from build123d import *

# Parameters (mm, degrees)
HEXAGONSOCKET_DEPTH = 1.1
CHAMFER_2_SIZE      = 0.2705
SKETCH_1_R          = 3.36
EXTRUDE_4_DEPTH     = 0.5
EXTRUDE_START       = 0.15
SKETCH_8_R          = 3.36
EXTRUDE_6_DEPTH     = 0.15
FILLET_5_R          = 0.2
CUT_EXTRUDE_START   = 3.14
SKETCH_6_R          = 1.5
CUT_EXTRUDE_1_DEPTH = 5.628101593
FILLET_6_R          = 0.15
CHAMFER_1_SIZE      = 0.15


with BuildPart() as part:
    # Sketch1 → Base (revolve)
    with BuildSketch(Plane.XY, mode=Mode.PRIVATE) as base_sk:
        Polygon((0, 0), (0, 3.36), (1.86, 1.5), (8, 1.5), (8, 0), align=None)
    revolve(base_sk.sketch.rotate(Axis((-0.587069181, 0, 0), (1, 0, 0)), 90), axis=Axis((-0.587069181, 0, 0), (1, 0, 0)))

    # Sketch2 → HexagonSocket (cut)
    with BuildSketch(Plane(origin=(0, 0, 0), x_dir=(0, 0, -1), z_dir=(1, 0, 0))):
        Polygon((1.154700538, 0), (0.577350269, 1), (-0.577350269, 1), (-1.154700538, 0), (-0.577350269, -1), (0.577350269, -1), align=None)
    extrude(amount=HEXAGONSOCKET_DEPTH, mode=Mode.SUBTRACT)

    # Sketch3 → Cut-Revolve1 (revolve, cut)
    with BuildSketch(Plane.XY, mode=Mode.PRIVATE) as cut_revolve1_sk:
        Polygon((1.1, 1), (1.677350269, 0), (1.1, 0), align=None)
    revolve(cut_revolve1_sk.sketch.rotate(Axis((-0.439109555, 0, 0), (1, 0, 0)), 90), axis=Axis((-0.439109555, 0, 0), (1, 0, 0)), mode=Mode.SUBTRACT)

    # Chamfer 2
    chamfer_2_edges = [part.edges().sort_by_distance(p)[0] for p in [
        (8, 0, -1.5),
    ]]
    chamfer(chamfer_2_edges, length=CHAMFER_2_SIZE)

    # 草图1 → 凸台-拉伸4 (add)
    with BuildSketch(Plane.ZY):
        Circle(SKETCH_1_R)
        Polygon((0.577350269, -1), (-0.577350269, -1), (-1.154700538, 0), (-0.577350269, 1), (0.577350269, 1), (1.154700538, 0), align=None, mode=Mode.SUBTRACT)
    extrude(amount=-EXTRUDE_4_DEPTH)

    # 草图5 → 旋转7 (revolve)
    with BuildSketch(Plane(origin=(0, 0, 0), x_dir=(1, 0, 0), z_dir=(0, 0.5000000000000003, 0.8660254037844386)), mode=Mode.PRIVATE) as revolve_7_sk:
        Polygon((2.632985321, -0.645763152), (0.5, -2.778748473), (0.5, -3.36), (2.632985321, -1.227014679), align=None)
    revolve(revolve_7_sk.sketch.rotate(Axis((1.86, 0, 0), (-1, 0, 0)), 60), axis=Axis((1.86, 0, 0), (-1, 0, 0)))

    # 草图8 → 凸台-拉伸6 (add)
    with BuildSketch(Plane.ZY.offset(EXTRUDE_START)):
        Circle(SKETCH_8_R)
        Polygon((0.577350269, -1), (-0.577350269, -1), (-1.154700538, 0), (-0.577350269, 1), (0.577350269, 1), (1.154700538, 0), align=None, mode=Mode.SUBTRACT)
    extrude(amount=-EXTRUDE_6_DEPTH)

    # 草图11 → 旋转8 (revolve)
    with BuildSketch(Plane(origin=(0, 0, 0), x_dir=(1, 0, 0), z_dir=(0, 0.5000000000000003, 0.8660254037844386)), mode=Mode.PRIVATE) as revolve_8_sk:
        Polygon((0.5, -3.36), (0.217401845, -3.642598155), (0, -3.86), (-0.15, -3.71), (-0.15, -3.36), align=None)
    revolve(revolve_8_sk.sketch.rotate(Axis((-0.15, 0, 0), (1, 0, 0)), 300), axis=Axis((-0.15, 0, 0), (1, 0, 0)))

    # 圆角5
    fillet_5_edges = [part.edges().sort_by_distance(p)[0] for p in [
        (0, 0, -3.86),
    ]]
    fillet(fillet_5_edges, radius=FILLET_5_R)

    # 草图6 → 切除-拉伸1 (cut, through all)
    with BuildSketch(Plane(origin=(2.36, 0, 0), x_dir=(0, 0, -1), z_dir=(1, 0, 0)).offset(CUT_EXTRUDE_START)):
        with Locations(Location((0, 0, 0), (0, 0, 180))):
            Circle(SKETCH_6_R)
    extrude(amount=CUT_EXTRUDE_1_DEPTH, mode=Mode.SUBTRACT)

    # 圆角6
    fillet_6_edges = [part.edges().sort_by_distance(p)[0] for p in [
        (2.36, 0, -1.5),
    ]]
    fillet(fillet_6_edges, radius=FILLET_6_R)

    # 倒角1
    chamfer_1_edges = [part.edges().sort_by_distance(p)[0] for p in [
        (5.5, 0, -1.5),
    ]]
    chamfer(chamfer_1_edges, length=CHAMFER_1_SIZE)


solid = part.part
Input: part model. Units: mm. Frame: model coordinates. Give positions to 0.01 mm unless a question says otherwise; leave off trailing zeros. Write each loop counter-clockwise with the first axis right and the second up, starting at its lowest first coordinate (ties: lowest second). Pieces come first, ordered by that corner, then holes. Notation, with made-up numbers: (-33.75, 78) -> (-27.75, 78) arc R8 cw to (-27.75, 84) -> close; hole circle Ø11 at (42.5, -9). An arc over 180 degrees is marked (long way). Use one line per item in the form item = value. Start each with the question number.
1) Draft query along Z for faces 1 (the flat face through (0.5, -1, 0)), 2 (the cylindrical face through (3.91, -0.45, 1.43)), 3 (the flat face through (5.5, 0, 0)). Return one class per face: pulls with the +Z half, pulls with the -Z half, needs draft (parallel to the pull), parting line crosses it, or undercut.
2) Pin query (flat end, axial travel): pin 1 (3 mm diameter, centred on x = 2.5, z = 1.5, fed in from -Y); pin 2 (2 mm diameter, centred on x = 4.5, y = -1.5, fed in from -Z); pin 3 (0.9 mm diameter, centred on x = 0.5, z = 0, fed in from -Y). Return the tip coordinate at first contact, or that it passes through.
3) Section query C-C on x = 4.8. Return the cut outline in (y, z), then the cut area to 3 significant figures.
4) Ray query, probe 1 along Z at (x, y) = (4.75, 0.25); probe 2 along X at (y, z) = (0.75, -2.25); probe 3 along Z at (x, y) = (2.85, -0.5). Return the intervals inside material, ascending. Write a range as from..to.
5) Section query A-A on x = 2.05. Return the cut outline in (y, z).
6) Section query B-B on x = 1.25. Return the cut outline in (y, z), then the cut area to 3 significant figures.
Outcome:
q1.face_1 = undercut
q1.face_2 = parting line crosses it
q1.face_3 = needs draft
q2.pin_1 = -2.59
q2.pin_2 = -1.41
q2.pin_3 = -3.77
q3.outline = circle Ø3 at (0, 0)
q3.area = 7.07 mm^2
q4.probe_1 = -1.48..1.48
q4.probe_2 = -0.15..1.49
q4.probe_3 = -1.41..1.41
q5.outline = circle Ø3.62 at (0, 0)
q6.outline = circle Ø5.22 at (0, 0); hole circle Ø1.48 at (0, 0)
q6.area = 19.7 mm^2
